from build123d import *

# Parameters (mm, degrees)
ESQUISSE1_W                  = 150
ESQUISSE1_H                  = 60
BOSS_EXTRU_1_DEPTH           = 8
ESQUISSE2_W                  = 80
ESQUISSE2_H                  = 60
ENL_V_MAT_EXTRU_1_DEPTH      = 3
ENL_V_MAT_EXTRU_2_DEPTH      = 162.632298752
ENL_V_MAT_EXTRU_2_DEPTH_BACK = 162.632298752
ESQUISSE3_R                  = 8
ESQUISSE4_W                  = 80
ESQUISSE4_H                  = 8
BOSS_EXTRU_2_DEPTH           = 3
CONG_1_R                     = 3
ESQUISSE5_R                  = 13.25
ENL_V_MAT_EXTRU_3_DEPTH      = 162.752897965


with BuildPart() as part:
    # Esquisse1 → Boss.-Extru.1 (new body)
    with BuildSketch(Plane.XY):
        with Locations((75, 30)):
            Rectangle(ESQUISSE1_W, ESQUISSE1_H)
    extrude(amount=BOSS_EXTRU_1_DEPTH)

    # Esquisse2 → Enlèv. mat.-Extru.1 (cut)
    with BuildSketch(Plane.XY.offset(8)):
        with Locations((75, 30)):
            Rectangle(ESQUISSE2_W, ESQUISSE2_H)
    extrude(amount=-ENL_V_MAT_EXTRU_1_DEPTH, mode=Mode.SUBTRACT)

    # Esquisse3 → Enlèv. mat.-Extru.2 (cut, two sides: drawn at the far end of the back side and taken through both)
    with BuildSketch(Plane.XY.offset(5).offset(-ENL_V_MAT_EXTRU_2_DEPTH_BACK)):
        with Locations((75, 24)):
            Circle(ESQUISSE3_R)
    extrude(amount=ENL_V_MAT_EXTRU_2_DEPTH + ENL_V_MAT_EXTRU_2_DEPTH_BACK, mode=Mode.SUBTRACT)

    # Esquisse4 → Boss.-Extru.2 (add)
    with BuildSketch(Plane.XY.offset(5)):
        with Locations((75, 4)):
            Rectangle(ESQUISSE4_W, ESQUISSE4_H)
    extrude(amount=BOSS_EXTRU_2_DEPTH)

    # Congé1
    cong_1_edges = [part.edges().sort_by_distance(p)[0] for p in [
        (35, 8, 6.5),
        (115, 8, 6.5),
    ]]
    fillet(cong_1_edges, radius=CONG_1_R)

    # Esquisse5 → Enlèv. mat.-Extru.3 (cut, through all)
    with BuildSketch(Plane.XY.offset(8)):
        with Locations((133.991524815, 23)):
            Circle(ESQUISSE5_R)
    extrude(amount=-ENL_V_MAT_EXTRU_3_DEPTH, mode=Mode.SUBTRACT)


solid = part.part
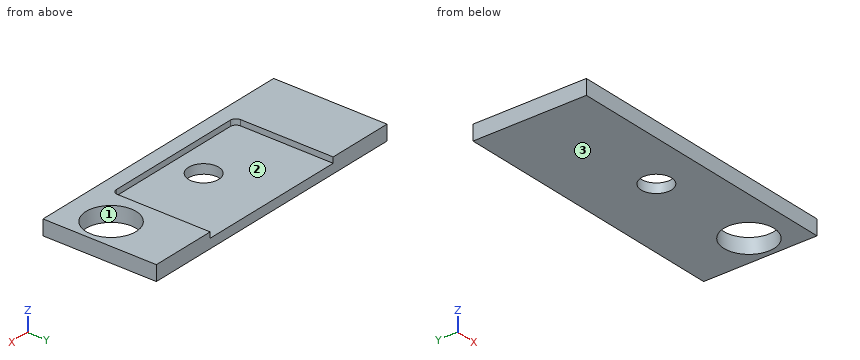
Geometry: final body of the model. Coordinates: model frame, mm. Face numbers are marked on the shaded views. Coordinates: 2 decimals unless noted, no trailing zeros. Order: outer loops, then holes, each group sorted by start corner. A loop starts at its lowest first (then second) coordinate and runs counter-clockwise, first axis right, second up.
(1) Section query D-D (x = 109). Return the cut outline in (y, z).
(2) Draft query along X for the marked faces 1, 2 and 3. Return one class per face: pulls with the +X half, pulls with the -X half, needs draft (parallel to the pull), parting line crosses it, or undercut.
(3) Section query B-B (z = 3.75). Return the cut outline in (x, y), plus the area to 3 significant figures.
(4) Section query C-C (y = 29.5). Return the cut outline in (x, z).
(5) Section query A-A (x = 75). Return the cut outline in (y, z).
(6) Material intervals for probe 1 along X at (y, z) = (28.5, 6.5); probe 2 along Y at (x, z) = (75, 1.55); probe 3 along X at (y, z) = (47, 7), sorted ascending.
(7) First-contact query: pin 1 (1.5 mm diameter, centred on x = 78, z = 6, fed in from +Y); pin 2 (6 mm diameter, centred on x = 81.5, y = 41.5, fed in from +Z). Flat tips, straight axial feed; report the tip coordinate or a pass-through.
Solution:
1. outline: (0, 0) - (60, 0) - (60, 5) - (8, 5) - (8, 8) - (0, 8) - close
2. face 1: undercut
2. face 2: undercut
2. face 3: needs draft
3. outline: (0, 0) - (150, 0) - (150, 60) - (0, 60) - close; hole circle Ø16 at (75, 24); hole circle Ø26.5 at (133.99, 23)
3. area: 8,250 mm2
4. outline: (0, 0) - (69.19, 0) - (69.19, 5) - (35, 5) - (35, 8) - (0, 8) - close; (80.81, 0) - (122.45, 0) - (122.45, 8) - (115, 8) - (115, 5) - (80.81, 5) - close; (145.54, 0) - (150, 0) - (150, 8) - (145.54, 8) - close
5. outline: (0, 0) - (16, 0) - (16, 5) - (8, 5) - (8, 8) - (0, 8) - close; (32, 0) - (60, 0) - (60, 5) - (32, 5) - close
6. probe 1: x = 0 to 35, 115 to 121.94, 146.05 to 150
6. probe 2: y = 0 to 16, 32 to 60
6. probe 3: x = 0 to 35, 115 to 150
7. pin 1: stops at y = 8
7. pin 2: stops at z = 5
